from build123d import *

# Parameters (mm, degrees)
SKETCH2_R                   = 6.5
BOSS_EXTRUDE1_DEPTH         = 10
M10X1_25_TAPPED_HOLE1_D     = 8.8
M10X1_25_TAPPED_HOLE1_DEPTH = 20
M10X1_25_TAPPED_HOLE1_TIP   = 2.643786724
SKETCH8_R                   = 14
CUT_EXTRUDE1_DEPTH          = 14
FILLET1_R                   = 1
CUT_EXTRUDE2_DEPTH          = 4
FILLET2_R                   = 2
FILLET2_OF_MIRROR1_R        = 2
CHAMFER1_SIZE               = 5


with BuildPart() as part:
    # Sketch2 → Boss-Extrude1 (new body, symmetric)
    with BuildSketch(Plane.XY):
        with BuildLine():
            Line((-18.33030278, 12), (-30, 12))
            Line((-30, 12), (-30, -38.93665036))
            ThreePointArc((-30, -38.93665036), (-30.363636327, -44.955902916), (-31.449256053, -50.887602716))
            Line((-31.449256053, -50.887602716), (-46, -110))
            Line((-46, -110), (-46, -125))
            Line((-46, -125), (46, -125))
            Line((46, -125), (46, -110))
            Line((46, -110), (31.449256053, -50.887602716))
            ThreePointArc((31.449256053, -50.887602716), (30.363636327, -44.955902916), (30, -38.93665036))
            Line((30, -38.93665036), (30, 12))
            Line((30, 12), (18.33030278, 12))
            ThreePointArc((18.33030278, 12), (16.33030278, 12.417424305), (14.664242224, 13.6))
            ThreePointArc((14.664242224, 13.6), (0, 20), (-14.664242224, 13.6))
            ThreePointArc((-14.664242224, 13.6), (-16.33030278, 12.417424305), (-18.33030278, 12))
        make_face()
        Circle(SKETCH2_R, mode=Mode.SUBTRACT)
    extrude(amount=BOSS_EXTRUDE1_DEPTH, both=True)

    # M10x1.25 Tapped Hole1
    with Locations(Plane(origin=(0, -125, 0), x_dir=(-1, 0, 0), z_dir=(0, -1, 0))):
        with Locations((30, 0), (-30, 0)):
            Hole(M10X1_25_TAPPED_HOLE1_D / 2, depth=M10X1_25_TAPPED_HOLE1_DEPTH)
            with Locations((0, 0, -(M10X1_25_TAPPED_HOLE1_DEPTH + M10X1_25_TAPPED_HOLE1_TIP / 2))):  # 118° drill point
                Cone(0, M10X1_25_TAPPED_HOLE1_D / 2, M10X1_25_TAPPED_HOLE1_TIP, mode=Mode.SUBTRACT)

    # Sketch8 → Cut-Extrude1 (cut)
    with BuildSketch(Plane.XY.offset(10)):
        Circle(SKETCH8_R)
    extrude(amount=-CUT_EXTRUDE1_DEPTH, mode=Mode.SUBTRACT)

    # Fillet1
    fillet1_edges = [part.edges().sort_by_distance(p)[0] for p in [
        (-14, 0, 10),
    ]]
    fillet(fillet1_edges, radius=FILLET1_R)

    # Sketch9 → Cut-Extrude2 (cut)
    with BuildSketch(Plane.XY.offset(10)):
        with BuildLine():
            Line((-30.703970126, -98.065082549), (-18, -46.455203914))
            Line((-18, -46.455203914), (-18, -30))
            ThreePointArc((-18, -30), (-16.535533906, -26.464466094), (-13, -25))
            Line((-13, -25), (13, -25))
            ThreePointArc((13, -25), (16.535533906, -26.464466094), (18, -30))
            Line((18, -30), (18, -46.455203914))
            Line((18, -46.455203914), (30.703970126, -98.065082549))
            ThreePointArc((30.703970126, -98.065082549), (29.784342096, -102.344373289), (25.848895731, -104.260177784))
            Line((25.848895731, -104.260177784), (-25.848895731, -104.260177784))
            ThreePointArc((-25.848895731, -104.260177784), (-29.784342096, -102.344373289), (-30.703970126, -98.065082549))
        make_face()
    cut_extrude2 = extrude(amount=-CUT_EXTRUDE2_DEPTH, mode=Mode.SUBTRACT)

    # Fillet2
    fillet2_edges = [part.edges().sort_by_distance(p)[0] for p in [
        (-18, -38.227601957, 6),
        (-16.535533906, -26.464466094, 6),
        (0, -25, 6),
        (16.535533906, -26.464466094, 6),
        (18, -38.227601957, 6),
        (24.351985063, -72.260143231, 6),
        (29.784342096, -102.344373289, 6),
        (0, -104.260177784, 6),
        (-29.784342096, -102.344373289, 6),
        (-24.351985063, -72.260143231, 6),
    ]]
    fillet(fillet2_edges, radius=FILLET2_R)

    # Mirror1: Cut-Extrude2 across plane
    add(cut_extrude2.mirror(Plane.XY), mode=Mode.SUBTRACT)

    # Fillet2 of Mirror1
    fillet2_of_mirror1_edges = [part.edges().sort_by_distance(p)[0] for p in [
        (-18, -38.227601957, -6),
        (-16.535533906, -26.464466094, -6),
        (0, -25, -6),
        (16.535533906, -26.464466094, -6),
        (18, -38.227601957, -6),
        (24.351985063, -72.260143231, -6),
        (29.784342096, -102.344373289, -6),
        (0, -104.260177784, -6),
        (-29.784342096, -102.344373289, -6),
        (-24.351985063, -72.260143231, -6),
    ]]
    fillet(fillet2_of_mirror1_edges, radius=FILLET2_OF_MIRROR1_R)

    # Chamfer1
    chamfer1_edges = [part.edges().sort_by_distance(p)[0] for p in [
        (30, 12, 0),
        (-30, 12, 0),
    ]]
    chamfer(chamfer1_edges, length=CHAMFER1_SIZE)


solid = part.part
Can you work these out from the model? Positions are in its coordinate system, mm. A direction names the side the tool comes from. Coordinates: 2 decimals unless noted, no trailing zeros. Write each loop counter-clockwise with the first axis right and the second up, starting at its lowest first coordinate (ties: lowest second). Pieces come first, ordered by that corner, then holes. Notation, with made-up numbers: (-13, 41.5) - (-1, 41.5) arc R32 cw to (-1, 76.5) - close; hole circle Ø6 at (-33, -15). An arc over 180 degrees is marked (long way). Return JSON: item names as keys, results as strings. Group by question number.
Item 1: Please list where these lines run through material, in increasing order: probe 1 along Z at (x, y) = (-30, -110.5); probe 2 along X at (y, z) = (-26, 8.75); probe 3 along X at (y, z) = (-28.5, -5.5).
Item 2: If we section it at B-B (x = 0): Write out the boundary of the cut face in (y, z).
Item 3: We'd pull the mould along X, two halves only. Please class faces 5 (the face through (-30.729, -102.815, -0.23)), 6 (the face through (16.357, 12.406, 0.14)), 7 (the face through (-1, -125, 0)): pulls with the +X half, pulls with the -X half, needs draft (parallel to the pull), parting line crosses it, or undercut.
Item 4: I'm going to push flat-ended pins straight in: pin 1 Ø2 at (y, z) = (5, -0.5) entering from -X; pin 2 Ø6 at (y, z) = (-43, -6.5) entering from -X; pin 3 Ø14 at (x, y) = (6, -0.5) entering from +Z. Where does each tip first touch, or does it pass through?
Item 5: If we section it at A-A (y = 0): Write out the boundary of the cut face in (x, z), then the cut area to 3 significant figures.
Item 6: Which directions (+Z, -Z, +X, -X, +Y, -Y) give clear straight access to the entire face, cutting with the end or side of a thin tool? Please do faces 1 (the face through (-22, 12, 0)), 2 (the face through (16, -26, -9)), 3 (the face through (24.263, -71.899, 9.014)), 4 (the face through (34.064, -114.86, 1.685)).
Return value:
{
 "1": {"probe 1": "z = -10 to -4.4, 4.4 to 10", "probe 2": "x = -30 to -16, 16 to 30", "probe 3": "x = -30 to 30"},
 "2": {"outline": "(-125, -10) - (-104.26, -10) - (-104.26, -8) arc R2 cw to (-102.26, -6) - (-27, -6) arc R2 cw to (-25, -8) - (-25, -10) - (-6.5, -10) - (-6.5, -4) - (-14, -4) - (-14, 9) arc R1 ccw to (-15, 10) - (-25, 10) - (-25, 8) arc R2 cw to (-27, 6) - (-102.26, 6) arc R2 cw to (-104.26, 8) - (-104.26, 10) - (-125, 10) - close; (6.5, -10) - (20, -10) - (20, 10) - (15, 10) arc R1 ccw to (14, 9) - (14, -4) - (6.5, -4) - close"},
 "3": {"face 5": "undercut", "face 6": "pulls with the +X half", "face 7": "needs draft"},
 "4": {"pin 1": "stops at x = -30", "pin 2": "stops at x = -30.5", "pin 3": "stops at z = -4"},
 "5": {"outline": "(-30, -10) - (-6.5, -10) - (-6.5, -4) - (-14, -4) - (-14, 9) arc R1 ccw to (-15, 10) - (-30, 10) - close; (6.5, -10) - (30, -10) - (30, 10) - (15, 10) arc R1 ccw to (14, 9) - (14, -4) - (6.5, -4) - close", "area": "730 mm^2"},
 "6": {"face 1": "+Z, -Z, -X, +Y", "face 2": "-Z", "face 3": "+Z", "face 4": "-Y"}
}
